Design review of the part built by this model. Coordinates are the model's own, in mm. A direction names the side the tool comes from. Coordinates: 2 decimals unless noted, no trailing zeros. Write each loop counter-clockwise with the first axis right and the second up, starting at its lowest first coordinate (ties: lowest second). Pieces come first, ordered by that corner, then holes.
Q1. The part is to be moulded in two halves that separate along Z. For faces 1 (the flat face through (19.9, -1.2, -75)), 2 (the cylindrical face through (5.57, -1.4, -59.16)), 3 (the flat face through (4, 11, -120)), say which applies: released by +Z, released by -Z, zero draft, split by the parting line, or undercut.
Q2. For pin 1 Ø6 at (y, z) = (5.5, -104.5) entering from +X; pin 2 Ø0.9 at (y, z) = (12.5, -99.5) entering from -X; pin 3 Ø1.5 at (x, z) = (1.5, -84.5) entering from +Y, all flat-tipped, find the tip position at first contact; note any pin that passes through.
Q3. Take a section at B-B, the plane z = -63.5. Write out the cut boundary in (x, y), plus the area to 3 significant figures.
Q4. Take a section at A-A, the plane x = 22.25. Write out the cut boundary in (y, z), plus the area to 3 significant figures.
Q5. For faces 4 (the cylindrical face through (11.48, 24.82, -60.21)), 5 (the cylindrical face through (26.55, -1.43, -97.18)), 6 (the flat face through (3, 13, -100)), list the 3-axis set-ups (+Z, -Z, +X, -X, +Y, -Y) from which the entire face can be reached by the end or side of a thin tool; tool diameter is ignored.
Q6. Take a section at C-C, the plane x = 16.5. Write out the cut boundary in (y, z), plus the area to 3 significant figures.
Q7. For L1, parallel to Y at x = 0.75, z = -100; L2, parallel to X at y = 13.25, z = -101.5; L3, parallel to X at y = 16, z = -82.5, list the stretches that pass through material, from the lowest coordinate up.
from build123d import *

# Parameters (mm, degrees)
SKETCH1_W        = 120
SKETCH1_H        = 25
BASE_DEPTH       = 5
CLIP_DEPTH       = 120
SKETCH3_R        = 1.5
SCREWHOLES_DEPTH = 3
ROUNDEDCORNERS_R = 1
SKETCH4_W        = 15.150992531
SKETCH4_H        = 29
FINGERGAP_DEPTH  = 15
FINGERGROOVE_R   = 5


with BuildPart() as part:
    # Sketch1 → Base (new body)
    with BuildSketch(Plane(origin=(0, 0, 0), x_dir=(0, 0, -1), z_dir=(1, 0, 0))):
        with Locations((60, 12.5)):
            Rectangle(SKETCH1_W, SKETCH1_H)
    extrude(amount=BASE_DEPTH)

    # Sketch2 → Clip (add)
    with BuildSketch(Plane.XY):
        with BuildLine():
            Line((25.150992531, 27), (7, 27))
            ThreePointArc((7, 27), (5.585786438, 26.414213562), (5, 25))
            Line((5, 25), (5, 12.5))
            ThreePointArc((5, 12.5), (12.740541767, 24.773008971), (27.150992531, 23.075468156))
            Line((27.150992531, 23.075468156), (27.150992531, 25))
            ThreePointArc((27.150992531, 25), (26.565206094, 26.414213562), (25.150992531, 27))
        make_face()
        with BuildLine():
            ThreePointArc((27.150992531, 1.924531844), (12.740541767, 0.226991029), (5, 12.5))
            Line((5, 12.5), (5, 0))
            ThreePointArc((5, 0), (5.585786438, -1.414213562), (7, -2))
            Line((7, -2), (25.150992531, -2))
            ThreePointArc((25.150992531, -2), (26.565206094, -1.414213562), (27.150992531, 0))
            Line((27.150992531, 0), (27.150992531, 1.924531844))
        make_face()
    extrude(amount=-CLIP_DEPTH)

    # Sketch3 → ScrewHoles (cut)
    with BuildSketch(Plane.ZY):
        with Locations((-100, 12.5)):
            Circle(SKETCH3_R)
        with Locations(Location((-20, 12.5, 0), (0, 0, 180))):
            Circle(SKETCH3_R)
    extrude(amount=-SCREWHOLES_DEPTH, mode=Mode.SUBTRACT)

    # RoundedCorners
    roundedcorners_edges = [part.edges().sort_by_distance(p)[0] for p in [
        (27.150992531, 23.075468156, -60),
        (27.150992531, 1.924531844, -60),
    ]]
    fillet(roundedcorners_edges, radius=ROUNDEDCORNERS_R)

    # Sketch4 → FingerGap (cut, symmetric)
    with BuildSketch(Plane(origin=(0, 0, -60), x_dir=(-1, 0, 0), z_dir=(0, 0, -1))):
        with Locations((-19.575496265, 12.5)):
            Rectangle(SKETCH4_W, SKETCH4_H)
    extrude(amount=FINGERGAP_DEPTH, both=True, mode=Mode.SUBTRACT)

    # FingerGroove
    # the kernel refuses this fillet: 5 mm, written as the material it takes off along each edge
    with BuildSketch(Plane(origin=(12, 0.608826803, -75), x_dir=(-0.8309099585253181, 0.5564069022068779, 0), z_dir=(0, 0, 1))) as fingergroove_piece_1:
        with BuildLine():
            CenterArc((2.68094623, 4.982639626), FINGERGROOVE_R, 213.807673482, 51.416397028)
            Line((-1.473603562, 2.200605115), (0, 0))
            ThreePointArc((0, 0), (1.132325116, 0.047220218), (2.264650232, 0))
        make_face()
    extrude(amount=30, mode=Mode.SUBTRACT)
    with BuildSketch(Plane(origin=(12, 24.391173197, -75), x_dir=(-0.8309099585253178, -0.5564069022068784, 0), z_dir=(0, 0, 1))) as fingergroove_piece_2:
        with BuildLine():
            CenterArc((2.68094623, -4.982639626), FINGERGROOVE_R, 94.77592949, 51.416397028)
            Line((-1.473603562, -2.200605115), (0, 0))
            ThreePointArc((0, 0), (1.132325116, -0.047220218), (2.264650232, 0))
        make_face()
    extrude(amount=30, mode=Mode.SUBTRACT)


solid = part.part
Responses:
1. face 1: undercut
1. face 2: zero draft
1. face 3: released by -Z
2. pin 1: stops at x = 9.38
2. pin 2: stops at x = 3
2. pin 3: stops at y = 25
3. outline: (0, 0) - (5, 0) arc R2 ccw to (7, -2) - (12, -2) arc R5 ccw to (10.12, 1.87) arc R13.6 cw to (10.12, 23.13) arc R5 ccw to (12, 27) - (7, 27) arc R2 ccw to (5, 25) - (0, 25) - close
3. area: 206 mm2
4. outline: (-2, -120) - (-0.6, -120) - (-0.6, -75) - (-2, -75) - close; (-2, -45) - (-0.6, -45) - (-0.6, 0) - (-2, 0) - close; (25.6, -120) - (27, -120) - (27, -75) - (25.6, -75) - close; (25.6, -45) - (27, -45) - (27, 0) - (25.6, 0) - close
4. area: 252 mm2
5. face 4: +X
5. face 5: +Z, -Z, +X, -Y
5. face 6: -X
6. outline: (-2, -120) - (-0.94, -120) - (-0.94, -75) - (-2, -75) - close; (-2, -45) - (-0.94, -45) - (-0.94, 0) - (-2, 0) - close; (25.94, -120) - (27, -120) - (27, -75) - (25.94, -75) - close; (25.94, -45) - (27, -45) - (27, 0) - (25.94, 0) - close
6. area: 191 mm2
7. L1: y = 0 to 11, 14 to 25
7. L2: x = 0 to 5.02
7. L3: x = 0 to 5.46
